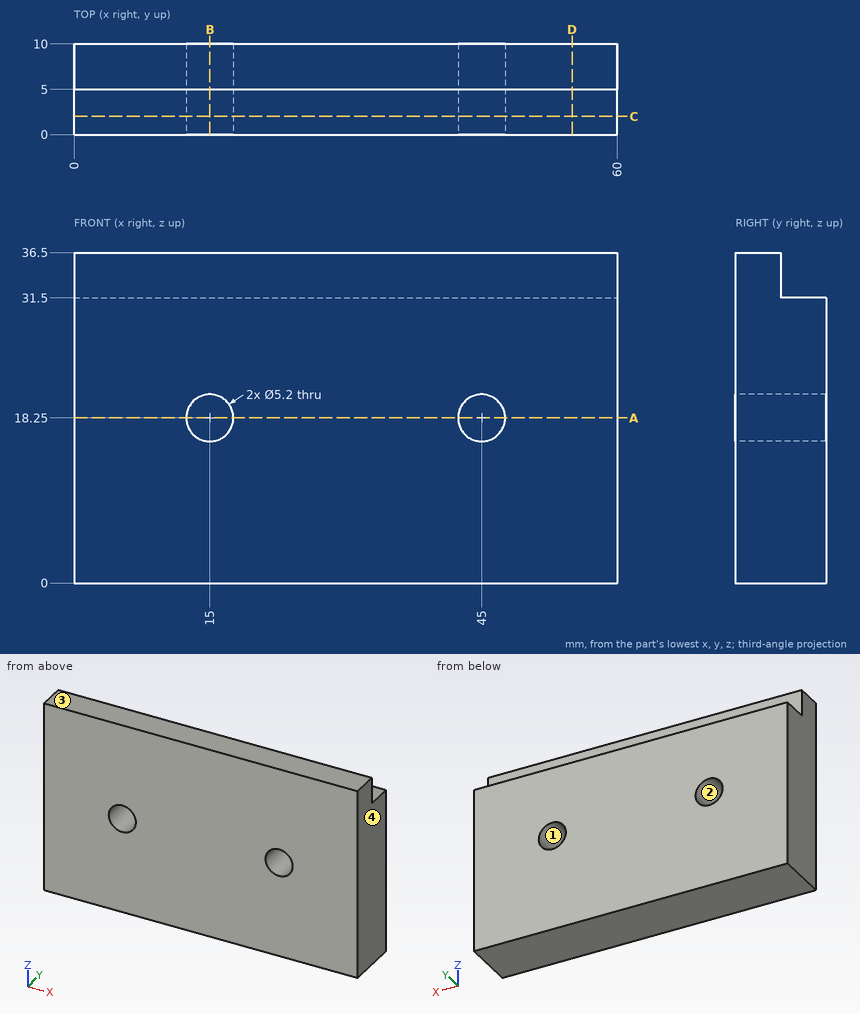
The drawing under review shows one solid part. Ordinate dimensions are in mm from its lowest x, y, z. Coordinates: 2 decimals unless noted, no trailing zeros. Write each loop counter-clockwise with the first axis right and the second up, starting at its lowest first coordinate (ties: lowest second). Pieces come first, ordered by that corner, then holes. Notation, with made-up numbers: (-7.5, -6) -> (49.5, -6) arc R15 cw to (49.5, 1) -> close; hole circle Ø3 at (70.25, 89.5). An arc over 180 degrees is marked (long way). One line per item, written item: value. Start each with the question number.
Q1. Add section B-B, the plane x = 15. Give the boundary of the cut face in (y, z).
Q2. The part is to be moulded in two halves that separate along Z. For the marked faces 1, 2, 3 and 4, say which applies: +Z half, -Z half, draft (parallel to the pull), parting line (faces both ways), or undercut.
Q3. Clearance check with flat-ended pins moving along their axes: P1, Ø2.5, axis at x = 28, y = 8.5, coming from the +Z side; P2, Ø4, axis at x = 36.5, z = 35, coming from the +Y side. State where each tip first meets the part, or that it passes through.
Q4. To check wall thickness, follow probe 1 along X at (y, z) = (3.75, 18.25); probe 2 along X at (y, z) = (1, 17); probe 3 along Z at (x, y) = (37.5, 6.75). State the ranges of each line that lie inside material, in increasing order.
Q5. Add section A-A, the plane z = 18.25. Give the boundary of the cut face in (x, y), then the cut area to 3 significant figures.
Q6. Add section C-C, the plane y = 2. Give the boundary of the cut face in (x, z).
Q7. Add section D-D, the plane x = 55. Give the boundary of the cut face in (y, z).
Response:
1. outline: (0, 0) -> (10, 0) -> (10, 15.65) -> (0, 15.65) -> close; (0, 20.85) -> (10, 20.85) -> (10, 31.5) -> (5, 31.5) -> (5, 36.5) -> (0, 36.5) -> close
2. face 1: undercut
2. face 2: undercut
2. face 3: +Z half
2. face 4: draft
3. P1: z = 31.5
3. P2: y = 5
4. probe 1: 0 to 12.4, 17.6 to 42.4, 47.6 to 60
4. probe 2: 0 to 12.72, 17.28 to 42.72, 47.28 to 60
4. probe 3: 0 to 31.5
5. outline: (0, 0) -> (12.4, 0) -> (12.4, 10) -> (0, 10) -> close; (17.6, 0) -> (42.4, 0) -> (42.4, 10) -> (17.6, 10) -> close; (47.6, 0) -> (60, 0) -> (60, 10) -> (47.6, 10) -> close
5. area: 496 mm²
6. outline: (0, 0) -> (60, 0) -> (60, 36.5) -> (0, 36.5) -> close; hole circle Ø5.2 at (15, 18.25); hole circle Ø5.2 at (45, 18.25)
7. outline: (0, 0) -> (10, 0) -> (10, 31.5) -> (5, 31.5) -> (5, 36.5) -> (0, 36.5) -> close
